```python
from build123d import *

# Parameters (mm, degrees)
F0_R     = 380
F1_DEPTH = 1750
F2_R     = 14
F3_DEPTH = 410
F4_R     = 40
F5_DEPTH = 60
F8_R     = 25
F9_DEPTH = 400


with BuildPart() as f1:
    # F0 (on Top) → F1 (new body)
    with BuildSketch(Plane.XY):
        Circle(F0_R)
    extrude(amount=F1_DEPTH)

    # F2 (on Front) → F3 (join)
    with BuildSketch(Plane.XZ):
        with Locations((0, 245)):
            Circle(F2_R)
        with Locations((0, 1340)):
            Circle(F2_R)
    extrude(amount=F3_DEPTH)

    # F4 (on face) → F5 (join)
    with BuildSketch(Plane.XY.offset(1750)):
        with Locations((-100, 0)):
            Circle(F4_R)
    extrude(amount=F5_DEPTH)

    # F8 (on face) → F9 (join)
    with BuildSketch(Plane(origin=(0, 0, 0), x_dir=(-0.939693, 0.34202, 0), z_dir=(0.34202, 0.939693, 0))):
        with Locations((0, 357)):
            Circle(F8_R)
    extrude(amount=-F9_DEPTH)


solid = f1.part
```
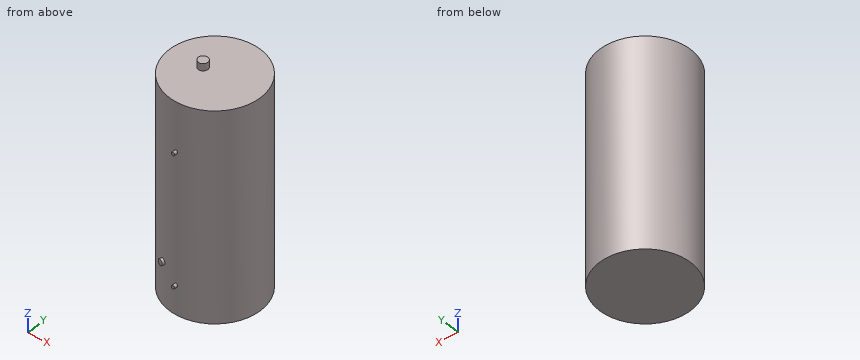
The listing builds one solid part. Answer for the finished solid, in the listing's coordinates (mm). Coordinates: 2 decimals unless noted, no trailing zeros. Write each loop counter-clockwise with the first axis right and the second up, starting at its lowest first coordinate (ties: lowest second). Pieces come first, ordered by that corner, then holes. Notation, with made-up numbers: (-11.75, -32) - (17.25, -32) arc R7 cw to (17.25, -28) - close; hole circle Ø11 at (12.5, -23). An arc over 180 degrees is marked (long way). One line per item, written item: value.
1) Each of these flat-tipped pins is pushed along its axis until it touches: pin 1 Ø3 at (y, z) = (248, 1418.5) entering from -X; pin 2 Ø2 at (x, z) = (81.5, 1472) entering from -Y; pin 3 Ø1.5 at (y, z) = (182.5, 774.5) entering from +X; pin 4 Ø1.5 at (x, y) = (121.5, -224.5) entering from -Z. Where does it stop, or does it pass through?
Geometry check:
pin 1: stops at x = -289.2
pin 2: stops at y = -371.38
pin 3: stops at x = 333.72
pin 4: stops at z = 0
2) Find section B-B (x = 39). Give the vertices of the cut face in (y, z).
Geometry check:
outline: (-377.99, 0) - (377.99, 0) - (377.99, 1750) - (-377.99, 1750) - close
3) Find section C-C (y = -222). Give the vertices of the cut face in (x, z).
Geometry check:
outline: (-308.41, 0) - (308.41, 0) - (308.41, 1750) - (-308.41, 1750) - close
4) Find section A-A (z = 829). Give the vertices of the cut face in (x, y).
Geometry check:
outline: circle Ø760 at (0, 0)
5) Consider line 1 along Z through (x, y) = (186.5, -60.5); line 2 along X through (y, z) = (-7, 1552.5); line 3 along X through (y, z) = (-161, 1021.5). Determine where each line is inside the solid, lowest interval first. Write a range as from..to.
Geometry check:
line 1: z = 0..1750
line 2: x = -379.94..379.94
line 3: x = -344.21..344.21
